Read the model definition and answer for the solid it produces. Units are mm, in the model's axes. A direction names the side the tool comes from. Give positions to 0.01 mm unless a question says otherwise; leave off trailing zeros. Order: outer loops, then holes, each group sorted by start corner. A loop starts at its lowest first (then second) coordinate and runs counter-clockwise, first axis right, second up. Notation, with made-up numbers: (-35, 27.25) - (12, 27.25) arc R15 cw to (12, 40.25) - close; hole circle Ø5 at (-17.75, 80.25). An arc over 180 degrees is marked (long way). Return JSON: item names as keys, results as strings.
Autodesk Inventor part; units mm, degrees
ref_plane "YZ Plane" through (0, 0, 0) normal (1, 0, 0) x (0, 1, 0)
ref_plane "XZ Plane" through (0, 0, 0) normal (0, 1, 0) x (-1, 0, 0)
ref_plane "XY Plane" through (0, 0, 0) normal (0, 0, 1) x (1, 0, 0)
sketch "Sketch1" plane through (0, 0, 0) normal (0, 1, 0) x (-1, 0, 0)
  line L0 (0, 0) -> (127, 0)
  line L1 (119.38, -9.525) -> (9.525, -9.525)
  line L2 (0, -9.525) -> (0, 0)
  arc A0 (0, -9.525) -> (9.525, -9.525) centre (4.7625, -10.16) ccw
  arc A1 (119.38, -9.525) -> (127, 0) centre (123.19, -4.7625) ccw
  circle A2 centre (123.19, -4.7625) radius 2.2479
  circle A3 centre (107.188, -4.7625) radius 2.2479
  circle A4 centre (89.6366, -4.7625) radius 1.9685
  circle A5 centre (79.8576, -4.7625) radius 1.9685
  circle A6 centre (70.0786, -4.7625) radius 1.9685
  circle A7 centre (60.2996, -4.7625) radius 1.9685
  circle A8 centre (50.5206, -4.7625) radius 1.9685
  circle A9 centre (40.7416, -4.7625) radius 1.9685
  circle A10 centre (30.9626, -4.7625) radius 1.9685
  circle A11 centre (21.1836, -4.7625) radius 1.9685
  dimension "d9" = 9.525
  dimension "d10" = 127
  dimension "d11" = 4.4958
  dimension "d12" = 4.4958
  dimension "d13" = 16.002
  dimension "d14" = 3.937
  dimension "d15" = 17.5514
  dimension "d18" = 9.779
extrude "Extrusion1" add sketch "Sketch1" along normal blind 3.175
sketch "Sketch2" plane through (0, 3.175, 0) normal (0, 1, 0) x (1, 0, 0)
  circle A0 centre (-40.7416, 4.7625) radius 1.9685 construction
  arc A1 (0, 9.525) -> (-9.525, 9.525) centre (-4.7625, 10.16) ccw construction
  line L0 (0, 0) -> (-6.35, 0)
  line L1 (-6.35, 0) -> (-6.35, 9.525)
  line L2 (-9.525, 9.525) -> (-6.35, 9.525)
  line L3 (0, 9.525) -> (0, 0)
  line L4 (-127, 0) -> (0, 0)
  line L5 (0, 0) -> (0, 9.525)
  arc A2 (0, 9.525) -> (-9.525, 9.525) centre (-4.7625, 10.16) ccw
  point P0 (-4.7625, 4.7625)
  dimension "d27" = 0
  dimension "d28" = 6.35
  dimension "d32" = 0
extrude "Extrusion2" add sketch "Sketch2" along normal blind 9.525
fillet "Fillet2" radius 3.175 1 edges at (0, 6.35, 0)
properties part number "CollectorArmRear"
Q1. Given pin 1 (2.5 mm diameter, centred on x = -79.86, z = -4.76, fed in from -Y); pin 2 (1.5 mm diameter, centred on x = -50, z = -7.5, fed in from +Y) (3 decimals); pin 3 (1 mm diameter, centred on x = -39.5, y = 2, fed in from -Z) (3 decimals); pin 4 (4 mm diameter, centred on y = 10.5, z = -7.5, fed in from +X), each flat-ended and moving along its own axis, determine where each tip first touches the part or whether it passes through.
Values:
{"pin 1": "passes through", "pin 2": "stops at y = 3.175", "pin 3": "stops at z = -9.525", "pin 4": "stops at x = 0"}
Q2. Consider L1, parallel to X at y = 11, z = -9; L2, parallel to Y at x = -53.5, z = -4.5 (3 decimals); L3, parallel to Z at x = -61, y = 3 (3 decimals). Determine where each line is inside the solid, lowest interval first.
Values:
{"L1": "x = -6.35 to 0", "L2": "y = 0 to 3.175", "L3": "z = -9.525 to -6.602, -2.923 to 0"}
Q3. A cutting plane is placed at A-A (x = -123.19). Write down the section's boundary in (y, z) (3 decimals), and give its area (3 significant figures).
Values:
{"outline": "(0, -10.861) - (3.175, -10.861) - (3.175, -7.01) - (0, -7.01) - close; (0, -2.515) - (3.175, -2.515) - (3.175, 0) - (0, 0) - close", "area": "20.2 mm²"}
Q4. For faces 1 (the flat face through (-60, 3, 0)), 2 (the flat face through (-65, 2, -9.525)), determine the directions among +Z, -Z, +X, -X, +Y, -Y from which every point of the face is accessible in a straight line to the end or side of a thin tool.
Values:
{"face 1": "+Z, +X, -X, +Y, -Y", "face 2": "-Z, +Y, -Y"}
Q5. Determine the mould class of faces 3 (the cylindrical face through (-68.112, 1.565, -4.849)), 4 (the flat face through (-6.35, 8, -5)), 5 (the flat face through (-8, 8, -9.525)) for opening direction Z: released by +Z, released by -Z, zero draft, split by the parting line, or undercut.
Values:
{"face 3": "undercut", "face 4": "zero draft", "face 5": "released by +Z"}
Q6. A cutting plane is placed at C-C (x = -95). Write down the section's boundary in (y, z) (3 decimals).
Values:
{"outline": "(0, -9.525) - (3.175, -9.525) - (3.175, 0) - (0, 0) - close"}
Q7. A cutting plane is placed at B-B (y = 1.5). Give the number of separate pieces and of enclosed holes in the cut face, and give its area (3 significant figures).
Values:
{"separate pieces": "1", "enclosed holes": "10", "area": "1,140 mm²"}
Q8. A cutting plane is placed at D-D (z = -13.5). Write down the section's boundary in (x, y), and give its area (3 significant figures).
Values:
{"outline": "(-8.22, 0) - (-1.31, 0) - (-1.31, 12.7) - (-8.22, 12.7) - close", "area": "87.7 mm²"}
